Autodesk Fusion 360 part; units mm, degrees
box "BoxPrimitive1" add length 15 width 39.5 height 2 placed x (0, 0, 1) y (1, 0, 0) z (0, 1, 0) at (0, 0, 0)
sketch "Sketch2" plane through (0, 0, 0) normal (1, 0, 0) x (0, 0, -1)
cylinder "CylinderPrimitive1" add diameter 2 height 39.5 placed x (0, 0, -1) y (0, 1, 0) z (1, 0, 0) at (0, 1.5, 1)
cylinder "CylinderPrimitive2" add diameter 2 height -39.5 placed x (0, 0, -1) y (0, 1, 0) z (1, 0, 0) at (39.5, 1.5, 7)
cylinder "CylinderPrimitive3" add diameter 2 height -39.5 placed x (0, 0, -1) y (0, 1, 0) z (1, 0, 0) at (39.5, 1.5, 13)
cylinder "CylinderPrimitive4" add diameter 2 height -15 placed x (0, 1, 0) y (1, 0, 0) z (0, 0, -1) at (2, 1.5, 0)
cylinder "CylinderPrimitive6" add diameter 2 height -15 placed x (0, 1, 0) y (1, 0, 0) z (0, 0, -1) at (14, 1.5, 0)
cylinder "CylinderPrimitive8" add diameter 2 height -15 placed x (0, 1, 0) y (1, 0, 0) z (0, 0, -1) at (26, 1.5, 0)
cylinder "CylinderPrimitive10" add diameter 2 height -15 placed x (0, 1, 0) y (1, 0, 0) z (0, 0, -1) at (38, 1.5, 0)
Can you work these out from the model? Positions are in its coordinate system, mm. A direction names the side the tool comes from. Give positions to 0.01 mm unless a question says otherwise; leave off trailing zeros. Order: outer loops, then holes, each group sorted by start corner. A loop starts at its lowest first (then second) coordinate and runs counter-clockwise, first axis right, second up. Notation, with made-up numbers: M 32,12 L 88,12 A26 cw 88,27 Z; hole C 7.5,75 d3. An arc over 180 degrees is marked long. One line per item, written item: value.
Item 1: Please list where these lines run through material, in increasing order: line 1 (Z direction, x = 4, y = 2.1); line 2 (Y direction, x = 31, z = 11.5); line 3 (X direction, y = 2.4, z = 8.25).
Verdict:
line 1: 0.2 to 1.8, 6.2 to 7.8, 12.2 to 13.8
line 2: 0 to 2
line 3: 1.56 to 2.44, 13.56 to 14.44, 25.56 to 26.44, 37.56 to 38.44
Item 2: If we section it at B-B on z = 2.5: Write out the boundary of the cut face in (x, y), and give its area (3 significant figures).
Verdict:
outline: M 0,0 L 39.5,0 L 39.5,2 L 38.87,2 A1 ccw 37.13,2 L 26.87,2 A1 ccw 25.13,2 L 14.87,2 A1 ccw 13.13,2 L 2.87,2 A1 ccw 1.13,2 L 0,2 Z
area: 81.5 mm2
Item 3: For faces 1 (the face through (38.9, 2.5, 1)), 2 (the face through (0.8, 2.5, 7)), 3 (the face through (26, 2.5, 14.2)), 4 (the face through (2, 2.5, 10)), 5 (the face through (0.6, 2, 14.4)), which set-ups out of +Z, -Z, +X, -X, +Y, -Y let a thin tool reach every point of the face, with its end or its side?
Verdict:
face 1: +X, +Y
face 2: -X, +Y
face 3: +Z, +Y
face 4: +Y
face 5: +Z, -X, +Y
Item 4: If we mould it in two halves opening along X, with no side actions, what happens to faces 6 (the face through (8, 2, 10)), 7 (the face through (0, 1, 8)), 8 (the face through (20, 0, 7))? For each: pulls with the +X half, pulls with the -X half, needs draft (parallel to the pull), parting line crosses it, or undercut.
Verdict:
face 6: undercut
face 7: pulls with the -X half
face 8: needs draft
Item 5: For pin 1 (0.7 mm diameter, centred on x = 39, z = 10.5, fed in from +Y); pin 2 (0.9 mm diameter, centred on x = 0.5, z = 14.5, fed in from +Y); pin 3 (3.5 mm diameter, centred on x = 33, z = 3.5, fed in from +Y), each with a flat end and sliding along its axis, tell me the tip position at first contact or that it passes through.
Verdict:
pin 1: y = 2.26
pin 2: y = 2
pin 3: y = 2.16
Item 6: If we section it at A-A on x = 11: Write out the boundary of the cut face in (y, z).
Verdict:
outline: M 0,0 L 2,0 L 2,0.13 A1 ccw 2,1.87 L 2,6.13 A1 ccw 2,7.87 L 2,12.13 A1 ccw 2,13.87 L 2,15 L 0,15 Z
Item 7: If we section it at C-C on z = 13.5: Write out the boundary of the cut face in (x, y).
Verdict:
outline: M 0,0 L 39.5,0 L 39.5,2.37 L 38.5,2.37 A1 ccw 37.5,2.37 L 26.5,2.37 A1 ccw 25.5,2.37 L 14.5,2.37 A1 ccw 13.5,2.37 L 2.5,2.37 A1 ccw 1.5,2.37 L 0,2.37 Z
